The listing builds one solid part. Answer for the finished solid, in the listing's coordinates (mm). A direction names the side the tool comes from. Coordinates: 2 decimals unless noted, no trailing zeros. Order: outer loops, then holes, each group sorted by start corner. A loop starts at its lowest first (then second) coordinate and runs counter-clockwise, first axis right, second up.
```python
from build123d import *

# Parameters (mm, degrees)
BOSS_EXTRUDE1_DEPTH     = 38
CUT_EXTRUDE8_DEPTH      = 119.084715353
CUT_EXTRUDE8_DEPTH_BACK = 38


with BuildPart() as part:
    # Sketch1 → Boss-Extrude1 (new body)
    with BuildSketch(Plane(origin=(0, 0, 0), x_dir=(1, 0, 0), z_dir=(0, 1, 0))):
        Polygon((-100, 50), (-100, 38), (-62, 0), (0, 0), (0, 50), align=None)
    extrude(amount=BOSS_EXTRUDE1_DEPTH)

    # Sketch2 → Cut-Extrude8 (cut, two sides: drawn at the far end of the back side and taken through both)
    with BuildSketch(Plane(origin=(0, 0, 0), x_dir=(0, 0, -1), z_dir=(1, 0, 0)).offset(-CUT_EXTRUDE8_DEPTH_BACK)):
        Polygon((139.275123153, 107.293505315), (38, 38), (0, 12), (-101.275123153, -57.293505315), (-239.862133784, 145.256740991), (0.688112523, 309.843751622), align=None)
    extrude(amount=CUT_EXTRUDE8_DEPTH + CUT_EXTRUDE8_DEPTH_BACK, mode=Mode.SUBTRACT)


solid = part.part
```
(1) Find section D-D (y = 23). Write down the section's boundary in (x, z), and give its area (3 significant figures).
(2) Each of these flat-tipped pins is pushed along its axis until it touches: pin 1 Ø8 at (y, z) = (13.5, -20.5) entering from -X; pin 2 Ø12 at (x, y) = (-88.5, 16.5) entering from +Z. Where does it stop, or does it pass through?
(3) Find section A-A (y = 4.5). Write down the section's boundary in (x, z), and give its area (3 significant figures).
(4) For faces 1 (the face through (-19, 25, -19)), 2 (the face through (-49, 19, -50)), determine the directions among +Z, -Z, +X, -X, +Y, -Y from which every point of the face is accessible in a straight line to the end or side of a thin tool.
(5) Consider line 1 (X direction, y = 22.5, z = -22); line 2 (X direction, y = 17.5, z = -32); line 3 (Z direction, x = -18, y = 36). Determine where each line is inside the solid, lowest interval first.
(6) Find section B-B (x = -26.5). Write down the section's boundary in (y, z).
(7) Find section C-C (z = -30.5). Write down the section's boundary in (x, y).
Findings below:
1. outline: (-100, -50) - (0, -50) - (0, -16.08) - (-38, -16.08) - (-38, 0) - (-62, 0) - (-100, -38) - close
1. area: 3,670 mm2
2. pin 1: stops at x = -86.5
2. pin 2: stops at z = -20.5
3. outline: (-100, -50) - (0, -50) - (0, 0) - (-62, 0) - (-100, -38) - close
3. area: 4,280 mm2
4. face 1: +Z, +X, +Y
4. face 2: -Z, +X, -X, +Y, -Y
5. line 1: x = -84 to 0
5. line 2: x = -94 to 0
5. line 3: z = -50 to -35.08
6. outline: (0, -50) - (38, -50) - (38, -38) - (12, 0) - (0, 0) - close
7. outline: (-92.5, 0) - (0, 0) - (0, 32.87) - (-38, 32.87) - (-38, 38) - (-92.5, 38) - close
